Geometry: final body of the model. Coordinates: model frame, mm. A direction names the side the tool comes from. Round coordinates to 2 decimals unless told otherwise and drop trailing zeros. Write each loop counter-clockwise with the first axis right and the second up, starting at its lowest first coordinate (ties: lowest second). Pieces come first, ordered by that corner, then holes. Notation, with made-up numbers: M 87.25,72.25 L 97.25,72.25 A27 cw 97.25,108.25 Z; hole C -32,46 d3. An arc over 180 degrees is marked long. Answer as CSV lines item,"result". Start each with the question number.
Q1. Section query B-B on z = 22. Output: boundary loops of the cut face in (x, y).
Q2. Section query C-C on x = 16.5. Output: boundary loops of the cut face in (y, z).
Q3. First-contact query: pin 1 (12 mm diameter, centred on y = 51.5, z = 21.5, fed in from -X). Flat tip, straight axial feed; report the tip coordinate or a pass-through.
Q4. Mould query, pull axis Z, two halves, no side actions, for faces 1 (the flat face through (15.36, 20, 28)), 2 (the cylindrical face through (16.51, 67.01, 2.85)), 3 (the flat face through (17, 45, 56)), 4 (the flat face through (17, 63.22, 28)). Classes: pulls with the +Z half, pulls with the -Z half, needs draft (parallel to the pull), parting line crosses it, or undercut.
Q5. Ray query, probe 1 along Z at (x, y) = (17.3, 35.5); probe 2 along Y at (x, z) = (16.4, 26.5); probe 3 along Z at (x, y) = (15.7, 63). Return the intervals inside material, ascending.
Q6. Section query D-D on y = 66.5. Output: boundary loops of the cut face in (x, z).
Q7. Reachability of faces 5 (the flat face through (17, 42, 49.1)), 6 (the cylindrical face through (16.546, 22.3, 53.972)) from +Z, -Z, +X, -X, +Y, -Y: full face, straight path, thin tool, end or side. Return the list, or none.
Q8. Section query A-A on y = 47.5. Output: boundary loops of the cut face in (x, z), and give its area (3 significant figures).
```python
from build123d import *

# Parameters (mm, degrees)
BOSS_EXTRUDE1_DEPTH = 56
SKETCH14_W          = 42.2
SKETCH14_H          = 42.2
CUT_EXTRUDE1_DEPTH  = 56
CHAMFER1_SIZE       = 3.5
FILLET1_R           = 10
SKETCH16_W          = 12.4
SKETCH16_H          = 23
CUT_EXTRUDE3_DEPTH  = 95.009532523
CUT_EXTRUDE4_REACH  = 93.39
SKETCH17_W          = 15.453545708
SKETCH17_H          = 18
FILLET4_R           = 15
CUT_EXTRUDE5_DEPTH  = 92.389771857


with BuildPart() as part:
    # Sketch1 → Boss-Extrude1 (new body)
    with BuildSketch(Plane.XY):
        with BuildLine():
            Line((13.02, -7.9417418), (17.7, -7.9417418))
            Line((17.7, -7.9417418), (17.7, 70.02))
            Line((17.7, 70.02), (-10.566443095, 70.02))
            Line((-10.566443095, 70.02), (-10.566443095, 13.02))
            Line((-10.566443095, 13.02), (-5.317126718, 13.02))
            Line((-5.317126718, 13.02), (-4.287512407, 13.02))
            ThreePointArc((-4.287512407, 13.02), (-3.319474451, 12.619025549), (-2.9185, 11.650987593))
            Line((-2.9185, 11.650987593), (-2.9185, 11.539212407))
            ThreePointArc((-2.9185, 11.539212407), (-3.319474451, 10.571174451), (-4.287512407, 10.1702))
            Line((-4.287512407, 10.1702), (-6.476788598, 10.1702))
            ThreePointArc((-6.476788598, 10.1702), (-7.136510935, 9.729114651), (-6.981020848, 8.950903446))
            Line((-6.981020848, 8.950903446), (-3.672257405, 5.649701928))
            ThreePointArc((-3.672257405, 5.649701928), (-2.746830644, 5.032499411), (-1.655778399, 4.8158))
            Line((-1.655778399, 4.8158), (1.655778399, 4.8158))
            ThreePointArc((1.655778399, 4.8158), (2.746830644, 5.032499411), (3.672257405, 5.649701928))
            Line((3.672257405, 5.649701928), (6.981020848, 8.950903446))
            ThreePointArc((6.981020848, 8.950903446), (7.136510935, 9.729114651), (6.476788598, 10.1702))
            Line((6.476788598, 10.1702), (4.287512407, 10.1702))
            ThreePointArc((4.287512407, 10.1702), (3.319474451, 10.571174451), (2.9185, 11.539212407))
            Line((2.9185, 11.539212407), (2.9185, 11.650987593))
            ThreePointArc((2.9185, 11.650987593), (3.319474451, 12.619025549), (4.287512407, 13.02))
            Line((4.287512407, 13.02), (6.332886163, 13.02))
            Line((6.332886163, 13.02), (10.562594215, 13.019824354))
            ThreePointArc((10.562594215, 13.019824354), (12.303594776, 12.313982883), (13.019956614, 10.577284622))
            Line((13.019956614, 10.577284622), (13.02, 4.287469289))
            ThreePointArc((13.02, 4.287469289), (12.619025549, 3.319431332), (11.650987593, 2.918456882))
            Line((11.650987593, 2.918456882), (11.539212407, 2.918456882))
            ThreePointArc((11.539212407, 2.918456882), (10.571174451, 3.319431332), (10.1702, 4.287469289))
            Line((10.1702, 4.287469289), (10.1702, 6.402089023))
            ThreePointArc((10.1702, 6.402089023), (9.733877283, 7.055496588), (8.963146507, 6.90287605))
            Line((8.963146507, 6.90287605), (5.667020993, 3.614283579))
            ThreePointArc((5.667020993, 3.614283579), (5.046449321, 2.687255303), (4.8285, 1.593185507))
            Line((4.8285, 1.593185507), (4.8285, -1.593185507))
            ThreePointArc((4.8285, -1.593185507), (5.046449321, -2.687255303), (5.667020993, -3.614283579))
            Line((5.667020993, -3.614283579), (8.963146507, -6.90287605))
            ThreePointArc((8.963146507, -6.90287605), (9.733877283, -7.055496588), (10.1702, -6.402089023))
            Line((10.1702, -6.402089023), (10.1702, -4.287469289))
            ThreePointArc((10.1702, -4.287469289), (10.571174451, -3.319431332), (11.539212407, -2.918456882))
            Line((11.539212407, -2.918456882), (11.650987593, -2.918456882))
            ThreePointArc((11.650987593, -2.918456882), (12.619025549, -3.319431332), (13.02, -4.287469289))
            Line((13.02, -4.287469289), (13.02, -5.3170836))
            Line((13.02, -5.3170836), (13.02, -7.9417418))
        make_face()
    extrude(amount=BOSS_EXTRUDE1_DEPTH)

    # Sketch14 → Cut-Extrude1 (cut)
    with BuildSketch(Plane(origin=(17.7, 0, 0), x_dir=(0, 0, -1), z_dir=(1, 0, 0))):
        with Locations((-28, 42.12)):
            Rectangle(SKETCH14_W, SKETCH14_H)
    extrude(amount=-CUT_EXTRUDE1_DEPTH, mode=Mode.SUBTRACT)

    # Chamfer1
    chamfer1_edges = [part.edges().sort_by_distance(p)[0] for p in [
        (3.566778452, 21.02, 49.1),
        (3.566778452, 63.22, 49.1),
        (3.566778452, 63.22, 6.9),
        (3.566778452, 21.02, 6.9),
    ]]
    chamfer(chamfer1_edges, length=CHAMFER1_SIZE)

    # Fillet1
    fillet1_edges = [part.edges().sort_by_distance(p)[0] for p in [
        (3.566778452, 70.02, 56),
        (3.566778452, 70.02, 0),
    ]]
    fillet(fillet1_edges, radius=FILLET1_R)

    # Sketch16 → Cut-Extrude3 (cut, through all)
    with BuildSketch(Plane(origin=(17.7, 0, 0), x_dir=(0, 0, -1), z_dir=(1, 0, 0))):
        with Locations((-49.8, 3.5582582)):
            Rectangle(SKETCH16_W, SKETCH16_H)
    extrude(amount=-CUT_EXTRUDE3_DEPTH, mode=Mode.SUBTRACT)

    # Sketch17 → Cut-Extrude4 (cut, up to next)
    with BuildSketch(Plane.XY.offset(56), mode=Mode.PRIVATE) as cut_extrude4_sk1:
        with Locations((-5.893215949, 42.12)):
            Rectangle(SKETCH17_W, SKETCH17_H)
    cut_extrude4_tool1 = extrude(cut_extrude4_sk1.sketch, amount=-CUT_EXTRUDE4_REACH, mode=Mode.PRIVATE) & part.part
    add(cut_extrude4_tool1.solids().sort_by_distance((-5.893216, 42.12, 56))[0], mode=Mode.SUBTRACT)

    # Fillet4
    # the kernel refuses this fillet: 15 mm, written as the material it takes off along each edge
    with BuildSketch(Plane(origin=(54.632370625, 15.0582582, 56), x_dir=(0, 1, 0), z_dir=(-1, 0, 0))) as fillet4_piece_1:
        with BuildLine():
            CenterArc((14.77294825, 15), FILLET4_R, 189.98168298, 80.01831702)
            Line((0, 12.4), (-0.295458965, 12.348))
            ThreePointArc((-0.295458965, 12.348), (-0.3, 6.2), (-0.3, 0))
            Line((-0.3, 0), (0, -0.3))
            Line((0, -0.3), (14.77294825, -0.3))
            Line((14.77294825, -0.3), (14.77294825, 0))
        make_face()
    extrude(amount=102.131184346, mode=Mode.SUBTRACT)

    # Sketch18 → Cut-Extrude5 (cut, through all)
    with BuildSketch(Plane(origin=(0, 0, 0), x_dir=(-1, 0, 0), z_dir=(0, 0, -1))):
        Polygon((-15.359697471, 16.914250509), (-37.368077548, 16.914250509), (-37.368077548, -12.201573967), (-15.359697471, -12.201573967), (14.082488106, -12.201573967), (14.082488106, 72.835801267), (-15.359697471, 72.835801267), align=None)
    extrude(amount=-CUT_EXTRUDE5_DEPTH, mode=Mode.SUBTRACT)


solid = part.part
```
Entries:
1,outline,"M 15.36,16.91 L 17.7,16.91 L 17.7,21.02 L 15.36,21.02 Z; M 15.36,63.22 L 17.7,63.22 L 17.7,70.02 L 15.36,70.02 Z"
2,outline,"M 16.91,0 L 60.02,0 A10 ccw 70.02,10 L 70.02,46 A10 ccw 60.02,56 L 29.83,56 A15 ccw 16.91,48.63 Z; hole M 21.02,10.4 L 24.52,6.9 L 59.72,6.9 L 63.22,10.4 L 63.22,45.6 L 59.72,49.1 L 24.52,49.1 L 21.02,45.6 Z"
3,pin 1,"passes through"
4,face 1,"needs draft"
4,face 2,"pulls with the -Z half"
4,face 3,"pulls with the +Z half"
4,face 4,"undercut"
5,probe 1,"z = 0 to 6.9, 49.1 to 56"
5,probe 2,"y = 16.91 to 21.02, 63.22 to 70.02"
5,probe 3,"z = 0.45 to 10.18, 45.82 to 55.55"
6,outline,"M 15.36,2.38 L 17.7,2.38 L 17.7,53.62 L 15.36,53.62 Z"
7,face 5,"+X, -X"
7,face 6,"+Z, +X, -X, -Y"
8,outline,"M 15.36,0 L 17.7,0 L 17.7,6.9 L 15.36,6.9 Z; M 15.36,49.1 L 17.7,49.1 L 17.7,56 L 15.36,56 Z"
8,area,"32.3 mm^2"
